from build123d import *

# Parameters (mm, degrees)
SKETCH2_W           = 100
SKETCH2_H           = 100
BOSS_EXTRUDE1_DEPTH = 60
SKETCH3_R           = 31
CUT_EXTRUDE1_DEPTH  = 30
FILLET1_R           = 10
SKETCH4_W           = 60
SKETCH4_H           = 100
SKETCH4_R           = 15
BOSS_EXTRUDE2_DEPTH = 10
SKETCH6_R           = 5
BOSS_EXTRUDE3_DEPTH = 30


with BuildPart() as part:
    # Sketch2 → Boss-Extrude1 (new body)
    with BuildSketch(Plane(origin=(0, 0, 0), x_dir=(0, 0, -1), z_dir=(1, 0, 0))):
        Rectangle(SKETCH2_W, SKETCH2_H)
    extrude(amount=BOSS_EXTRUDE1_DEPTH)

    # Sketch3 → Cut-Extrude1 (cut)
    with BuildSketch(Plane.ZY):
        Circle(SKETCH3_R)
    extrude(amount=-CUT_EXTRUDE1_DEPTH, mode=Mode.SUBTRACT)

    # Fillet1
    fillet1_edges = [part.edges().sort_by_distance(p)[0] for p in [
        (30, -50, -50),
        (30, -50, 50),
    ]]
    fillet(fillet1_edges, radius=FILLET1_R)

    # Sketch4 → Boss-Extrude2 (add)
    with BuildSketch(Plane(origin=(0, 50, 0), x_dir=(1, 0, 0), z_dir=(0, 1, 0))):
        with Locations((30, 0)):
            Rectangle(SKETCH4_W, SKETCH4_H)
        with Locations(Location((30, 25, 0), (0, 0, 270))):
            Circle(SKETCH4_R, mode=Mode.SUBTRACT)
        with Locations(Location((30, -25, 0), (0, 0, 270))):
            Circle(SKETCH4_R, mode=Mode.SUBTRACT)
    extrude(amount=BOSS_EXTRUDE2_DEPTH)

    # Sketch6 → Boss-Extrude3 (add)
    with BuildSketch(Plane(origin=(60, 0, 0), x_dir=(0, 0, -1), z_dir=(1, 0, 0))):
        with BuildLine():
            Line((-50, 33.916521486), (-50, -13.916521486))
            ThreePointArc((-50, -13.916521486), (-53.168239134, -5.792483082), (-61, -1.958260743))
            ThreePointArc((-61, -1.958260743), (-72, 10), (-61, 21.958260743))
            ThreePointArc((-61, 21.958260743), (-53.168239134, 25.792483082), (-50, 33.916521486))
        make_face()
        with Locations((-60, 10)):
            Circle(SKETCH6_R, mode=Mode.SUBTRACT)
    boss_extrude3 = extrude(amount=-BOSS_EXTRUDE3_DEPTH)

    # Mirror1: Boss-Extrude3 across plane
    add(boss_extrude3.mirror(Plane(origin=(0, 0, 0), x_dir=(1, 0, 0), z_dir=(0, 0, -1))))


solid = part.part
Build history of the part. All positions in model axes, mm. A direction names the side the tool comes from. Coordinates: 2 decimals unless noted, no trailing zeros. Order: outer loops, then holes, each group sorted by start corner. A loop starts at its lowest first (then second) coordinate and runs counter-clockwise, first axis right, second up. Notation, with made-up numbers: (-27, -38.5) - (26, -38.5) arc R19 cw to (26, -4.5) - close; hole circle Ø2 at (-25.5, -7). An arc over 180 degrees is marked (long way). Write item = value, one per line. Start each with the question number.
1) Two-plate mould, pull along Z, no slides. Class faces 4 (the face through (30, 60, -1)), 5 (the face through (30, 50, 25)), 6 (the face through (30.42, -46.99, 47.15)): pulls with the +Z half, pulls with the -Z half, needs draft (parallel to the pull), parting line crosses it, or undercut.
2) 3-axis set-ups, long thin cutter, end or side, ignore diameter. For faces 1 (the face through (30, 5, -58)), 2 (the face through (42.65, 54.93, 33.06)), 3 (the face through (14.79, 30.736, -4.036)): which of +Z, -Z, +X, -X, +Y, -Y reach the whole face in a straight line?
3) Wall check: line 1 along Y through (x, z) = (11, 0); line 2 along X through (y, z) = (57.5, -25); line 3 along Z through (x, y) = (26.5, 53). Give the ranges that are in metal, low to high. Write a range as from..to.
4) Saw through at D-D on z = 0. Write the cut outline in (x, y), then the cut area to 3 significant figures.
5) Flat gauge pins, fed straight in: pin 1 Ø4 at (y, z) = (9.5, 55) entering from -X; pin 2 Ø10 at (x, y) = (16, 20) entering from +Z; pin 3 Ø9 at (x, z) = (30.5, 19.5) entering from +Y; pin 4 Ø6 at (y, z) = (10, 60) entering from -X. Where does each tip first touch, or does it go through?
6) Saw through at B-B on z = -58. Write the cut outline in (x, y).
7) Saw through at A-A on x = 7.5. Write the cut outline in (y, z), then the cut area to 3 significant figures.
8) Saw through at C-C on y = 10. Write the cut outline in (x, z).
From the geometry:
q1.face_4 = needs draft
q1.face_5 = undercut
q1.face_6 = pulls with the +Z half
q2.face_1 = -Z, -X, +Y, -Y
q2.face_2 = +Y
q2.face_3 = -X
q3.line_1 = -50..-31, 31..60
q3.line_2 = 0..15, 45..60
q3.line_3 = -50..-39.59, -10.41..10.41, 39.59..50
q4.outline = (0, -50) - (60, -50) - (60, 60) - (0, 60) - (0, 31) - (30, 31) - (30, -31) - (0, -31) - close
q4.area = 4,740 mm^2
q5.pin_1 = 30
q5.pin_2 = 50
q5.pin_3 = 50
q5.pin_4 = through
q6.outline = (30, -2.6) - (60, -2.6) - (60, 5.42) - (30, 5.42) - close; (30, 14.58) - (60, 14.58) - (60, 22.6) - (30, 22.6) - close
q7.outline = (-50, -40) arc R10 ccw to (-40, -50) - (60, -50) - (60, 50) - (-40, 50) arc R10 ccw to (-50, 40) - close; hole circle Ø62 at (0, 0)
q7.area = 7,940 mm^2
q8.outline = (0, -50) - (30, -50) - (30, -55) - (60, -55) - (60, 55) - (30, 55) - (30, 50) - (0, 50) - (0, 29.34) - (30, 29.34) - (30, -29.34) - (0, -29.34) - close; (30, -72) - (60, -72) - (60, -65) - (30, -65) - close; (30, 65) - (60, 65) - (60, 72) - (30, 72) - close
